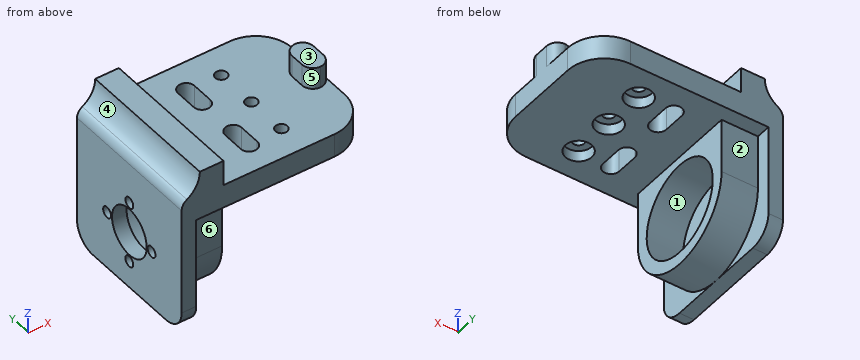
from build123d import *

# Parameters (mm, degrees)
ESBO_O1_W                  = 85
ESBO_O1_H                  = 40
RESSALTO_EXTRUS_O1_DEPTH   = 6.5
ESBO_O2_W                  = 11.5
ESBO_O2_H                  = 40
RESSALTO_EXTRUS_O2_DEPTH   = 7
CORTE_EXTRUS_O1_DEPTH      = 55.30469593
CORTE_EXTRUS_O1_DEPTH_BACK = 55.30469593
ESBO_O3_R                  = 1.625
ESBO_O6_R                  = 3.625
CORTE_EXTRUS_O3_DEPTH      = 3
ESBO_O7_W                  = 4
ESBO_O7_H                  = 40
RESSALTO_EXTRUS_O4_DEPTH   = 31
ESBO_O8_R                  = 12.625
RESSALTO_EXTRUS_O8_DEPTH   = 10
CORTE_EXTRUS_O4_DEPTH      = 90.0056178
CORTE_EXTRUS_O4_DEPTH_BACK = 90.0056178
ESBO_O10_R                 = 6.625
ESBO_O10_R_2               = 1.5
FILETE1_R                  = 6
CORTE_EXTRUS_O5_DEPTH      = 40
FILETE3_R                  = 3
CORTE_EXTRUS_O7_DEPTH      = 66.622023742
CORTE_EXTRUS_O7_DEPTH_BACK = 66.622023742
ESBO_O14_W                 = 5.875
ESBO_O14_H                 = 9.75
RESSALTO_EXTRUS_O9_DEPTH   = 6
FILETE4_R                  = 3
CORTE_EXTRUS_O8_DEPTH      = 66.622023742
CORTE_EXTRUS_O8_DEPTH_BACK = 66.622023742
ESBO_O15_W                 = 33.0625
ESBO_O15_H                 = 40
FILETE5_R                  = 10


with BuildPart() as part:
    # Esboço1 → Ressalto-extrusão1 (new body)
    with BuildSketch(Plane.XY):
        with Locations((-7.5, 0)):
            Rectangle(ESBO_O1_W, ESBO_O1_H)
    extrude(amount=RESSALTO_EXTRUS_O1_DEPTH)

    # Esboço2 → Ressalto-extrusão2 (add)
    with BuildSketch(Plane.XY.offset(6.5)):
        with Locations((-44.25, 0)):
            Rectangle(ESBO_O2_W, ESBO_O2_H)
    extrude(amount=RESSALTO_EXTRUS_O2_DEPTH)

    # Esboço3 → Corte-extrusão1 (cut, two sides: drawn at the far end of the back side and taken through both)
    with BuildSketch(Plane.XY.offset(6.5).offset(-CORTE_EXTRUS_O1_DEPTH_BACK)):
        with Locations((-16.5, -11.5)):
            Circle(ESBO_O3_R)
        with Locations((-16.5, 0)):
            Circle(ESBO_O3_R)
        with Locations((-16.5, 11.5)):
            Circle(ESBO_O3_R)
    extrude(amount=CORTE_EXTRUS_O1_DEPTH + CORTE_EXTRUS_O1_DEPTH_BACK, mode=Mode.SUBTRACT)

    # Esboço6 → Corte-extrusão3 (cut)
    with BuildSketch(Plane(origin=(0, 0, 0), x_dir=(-1, 0, 0), z_dir=(0, 0, -1))):
        with Locations((16.5, -11.5)):
            Circle(ESBO_O6_R)
        with Locations((16.5, 0)):
            Circle(ESBO_O6_R)
        with Locations((16.5, 11.5)):
            Circle(ESBO_O6_R)
    extrude(amount=-CORTE_EXTRUS_O3_DEPTH, mode=Mode.SUBTRACT)

    # Esboço7 → Ressalto-extrusão4 (add)
    with BuildSketch(Plane(origin=(0, 0, 0), x_dir=(-1, 0, 0), z_dir=(0, 0, -1))):
        with Locations((48, 0)):
            Rectangle(ESBO_O7_W, ESBO_O7_H)
    extrude(amount=RESSALTO_EXTRUS_O4_DEPTH)

    # Esboço8 → Ressalto-extrusão8 (add)
    with BuildSketch(Plane(origin=(-46, 0, 0), x_dir=(0, 0, -1), z_dir=(1, 0, 0))):
        with BuildLine():
            Line((15, -16), (0, -16))
            Line((0, -16), (0, 16))
            Line((0, 16), (15, 16))
            ThreePointArc((15, 16), (31, 0), (15, -16))
        make_face()
        with Locations((15, 0)):
            Circle(ESBO_O8_R, mode=Mode.SUBTRACT)
    extrude(amount=RESSALTO_EXTRUS_O8_DEPTH)

    # Esboço10 → Corte-extrusão4 (cut, two sides: drawn at the far end of the back side and taken through both)
    with BuildSketch(Plane(origin=(-46, 0, 0), x_dir=(0, 0, -1), z_dir=(1, 0, 0)).offset(-CORTE_EXTRUS_O4_DEPTH_BACK)):
        with Locations((15, 0)):
            Circle(ESBO_O10_R)
        with Locations((15, -8.5)):
            Circle(ESBO_O10_R_2)
        with Locations((6.5, 0)):
            Circle(ESBO_O10_R_2)
        with Locations((15, 8.5)):
            Circle(ESBO_O10_R_2)
        with Locations((23.5, 0)):
            Circle(ESBO_O10_R_2)
    extrude(amount=CORTE_EXTRUS_O4_DEPTH + CORTE_EXTRUS_O4_DEPTH_BACK, mode=Mode.SUBTRACT)

    # Filete1
    filete1_edges = [part.edges().sort_by_distance(p)[0] for p in [
        (-48, 20, -31),
        (-48, -20, -31),
    ]]
    fillet(filete1_edges, radius=FILETE1_R)

    # Esboço11 → Corte-extrusão5 (cut)
    with BuildSketch(Plane(origin=(0, 20, 0), x_dir=(1, 0, 0), z_dir=(0, 1, 0))):
        with BuildLine():
            Line((-50, -6.5), (-50, -13.5))
            Line((-50, -13.5), (-45, -13.5))
            ThreePointArc((-45, -13.5), (-46.378372313, -9.198837366), (-50, -6.5))
        make_face()
    extrude(amount=-CORTE_EXTRUS_O5_DEPTH, mode=Mode.SUBTRACT)

    # Filete3
    filete3_edges = [part.edges().sort_by_distance(p)[0] for p in [
        (-50, 0, 6.5),
    ]]
    fillet(filete3_edges, radius=FILETE3_R)

    # Esboço13 → Corte-extrusão7 (cut, two sides: drawn at the far end of the back side and taken through both)
    with BuildSketch(Plane.XY.offset(6.5).offset(-CORTE_EXTRUS_O7_DEPTH_BACK)):
        with BuildLine():
            Line((-28, -6), (-28, -12))
            ThreePointArc((-28, -12), (-25.75, -14.25), (-23.5, -12))
            Line((-23.5, -12), (-23.5, -6))
            ThreePointArc((-23.5, -6), (-25.75, -3.75), (-28, -6))
        make_face()
        with BuildLine():
            Line((-23.5, 6), (-23.5, 12))
            ThreePointArc((-23.5, 12), (-25.75, 14.25), (-28, 12))
            Line((-28, 12), (-28, 6))
            ThreePointArc((-28, 6), (-25.75, 3.75), (-23.5, 6))
        make_face()
    extrude(amount=CORTE_EXTRUS_O7_DEPTH + CORTE_EXTRUS_O7_DEPTH_BACK, mode=Mode.SUBTRACT)

    # Esboço14 → Ressalto-extrusão9 (add)
    with BuildSketch(Plane.XY.offset(6.5)):
        with Locations((-1, 0)):
            Rectangle(ESBO_O14_W, ESBO_O14_H)
    extrude(amount=RESSALTO_EXTRUS_O9_DEPTH)

    # Filete4
    # the kernel refuses this fillet: 3 mm, written as the material it takes off along each edge
    with BuildSketch(Plane(origin=(-3.9375, 4.875, 6.5), x_dir=(0, -1, 0), z_dir=(0, 0, 1)), Plane(origin=(-3.9375, -4.875, 6.5), x_dir=(1, 0, 0), z_dir=(0, 0, 1)), Plane(origin=(1.9375, 4.875, 6.5), x_dir=(-1, 0, 0), z_dir=(0, 0, 1))) as filete4_piece_1:
        with BuildLine():
            CenterArc((FILETE4_R, FILETE4_R), FILETE4_R, 180, 90)
            Line((0, FILETE4_R), (0, 0))
            Line((0, 0), (FILETE4_R, 0))
        make_face()
    extrude(amount=13.5, mode=Mode.SUBTRACT)
    with BuildSketch(Plane(origin=(1.9375, -4.875, 6.5), x_dir=(-1, 0, 0), z_dir=(0, 0, 1))) as filete4_piece_2:
        with BuildLine():
            CenterArc((FILETE4_R, -FILETE4_R), FILETE4_R, 90, 90)
            Line((0, -FILETE4_R), (0, 0))
            Line((0, 0), (FILETE4_R, 0))
        make_face()
    extrude(amount=13.5, mode=Mode.SUBTRACT)

    # Esboço15 → Corte-extrusão8 (cut, two sides: drawn at the far end of the back side and taken through both)
    with BuildSketch(Plane.XY.offset(6.5).offset(-CORTE_EXTRUS_O8_DEPTH_BACK)):
        with Locations((18.46875, 0)):
            Rectangle(ESBO_O15_W, ESBO_O15_H)
    extrude(amount=CORTE_EXTRUS_O8_DEPTH + CORTE_EXTRUS_O8_DEPTH_BACK, mode=Mode.SUBTRACT)

    # Filete5
    filete5_edges = [part.edges().sort_by_distance(p)[0] for p in [
        (1.9375, 20, 3.25),
        (1.9375, -20, 3.25),
    ]]
    fillet(filete5_edges, radius=FILETE5_R)


solid = part.part
Verification items for the finished model (mm, model axes). Face numbers are marked on the shaded views. A direction names the side the tool comes from. Round coordinates to 2 decimals unless told otherwise and drop trailing zeros. Loops run counter-clockwise (first coordinate to the right, second up) from the corner with the lowest first, then second, coordinate; pieces in that order, holes last. Notation, with made-up numbers: (88, 17) - (134, 17) arc R29 cw to (134, 40) - close; hole circle Ø11 at (36, 14). An arc over 180 degrees is marked (long way). Answer in a Markdown table with one row per item. Add a question column.
Q1. Material ranges on line 1 (Y direction, x = -16.5, z = 5.35) (3 decimals); line 2 (Y direction, x = -16.5, z = 1) (3 decimals); line 3 (Y direction, x = -39.25, z = -15) (3 decimals), recorded low to high.
Q2. Section check B-B on z = -9.5. Enter the section's corners in (x, y), plus the area to 3 significant figures.
Q3. Section check A-A on x = -16.5. Enter the section's corners in (y, z) (3 decimals), plus the area to 3 significant figures.
Q4. Section check D-D on y = -17. Enter the section's corners in (x, z).
Q5. Section check C-C on x = -25.75. Enter the section's corners in (y, z), plus the area to 4 significant figures.
Q6. Release check for a two-part mould opening along X. For the marked faces 4, 5 and 6 record: pulls with the +X half, pulls with the -X half, needs draft (parallel to the pull), parting line crosses it, or undercut.
Q7. Tool access check on the marked faces 1, 2 and 3. Record the directions out of +Z, -Z, +X, -X, +Y, -Y that give a thin tool (end or side, any length) a straight path to the whole face; none if there is none.
Q8. Gauge pin test, flat ends, axial feed: pin 1 (3 mm diameter, centred on x = -39, z = -10, fed in from -Y); pin 2 (3 mm diameter, centred on y = 1, z = 9, fed in from -X); pin 3 (3.5 mm diameter, centred on x = -16.5, y = 0, fed in from +Z); pin 4 (8 mm diameter, centred on x = -43, z = -4.5, fed in from +Y). Record the tip position at first contact, or that the pin passes through.
Found:
| question | item | result |
|---|---|---|
| 1 | line 1 | y = -20 to -13.125, -9.875 to -1.625, 1.625 to 9.875, 13.125 to 20 |
| 1 | line 2 | y = -20 to -15.125, -7.875 to -3.625, 3.625 to 7.875, 15.125 to 20 |
| 1 | line 3 | y = -16 to -12.625, 12.625 to 16 |
| 2 | outline | (-50, -20) - (-46, -20) - (-46, -16) - (-36, -16) - (-36, -11.36) - (-46, -11.36) - (-46, -3.69) - (-50, -3.69) - close; (-50, 3.69) - (-46, 3.69) - (-46, 11.36) - (-36, 11.36) - (-36, 16) - (-46, 16) - (-46, 20) - (-50, 20) - close |
| 2 | area | 223 mm² |
| 3 | outline | (-20, 0) - (-15.125, 0) - (-15.125, 3) - (-13.125, 3) - (-13.125, 6.5) - (-20, 6.5) - close; (-9.875, 3) - (-7.875, 3) - (-7.875, 0) - (-3.625, 0) - (-3.625, 3) - (-1.625, 3) - (-1.625, 6.5) - (-9.875, 6.5) - close; (1.625, 3) - (3.625, 3) - (3.625, 0) - (7.875, 0) - (7.875, 3) - (9.875, 3) - (9.875, 6.5) - (1.625, 6.5) - close; (13.125, 3) - (15.125, 3) - (15.125, 0) - (20, 0) - (20, 6.5) - (13.125, 6.5) - close |
| 3 | area | 161 mm² |
| 4 | outline | (-50, -30.2) - (-46, -30.2) - (-46, 0) - (-0.92, 0) - (-0.92, 6.5) - (-38.5, 6.5) - (-38.5, 13.5) - (-45, 13.5) arc R7.4 cw to (-48.56, 7.18) arc R3 ccw to (-50, 4.61) - close |
| 5 | outline | (-20, 0) - (-14.25, 0) - (-14.25, 6.5) - (-20, 6.5) - close; (-3.75, 0) - (3.75, 0) - (3.75, 6.5) - (-3.75, 6.5) - close; (14.25, 0) - (20, 0) - (20, 6.5) - (14.25, 6.5) - close |
| 5 | area | 123.5 mm² |
| 6 | face 4 | pulls with the -X half |
| 6 | face 5 | undercut |
| 6 | face 6 | needs draft |
| 7 | face 1 | +X |
| 7 | face 2 | -Z, +X, +Y |
| 7 | face 3 | +Z, +X, +Y, -Y |
| 8 | pin 1 | stops at y = -16 |
| 8 | pin 2 | stops at x = -48.07 |
| 8 | pin 3 | stops at z = 6.5 |
| 8 | pin 4 | stops at y = 20 |
